from build123d import *

# Parameters (mm, degrees)
SKETCH_1_R      = 12.5
EXTRUDE_1_DEPTH = 4


with BuildPart() as part:
    # 草图1 → 凸台-拉伸1 (new, symmetric)
    with BuildSketch(Plane(origin=(0, 0, 0), x_dir=(1, 0, 0), z_dir=(0, 1, 0))):
        Polygon((-75, 99.709683748), (75, 99.709683748), (119.42074844, 45.609802898), (85, -37.547951261), (-85, -37.547951261), (-119.42074844, 45.609802898), align=None)
        with Locations(Location((-95.730005712, 40.398538957, 0), (0, 0, 270))):
            Circle(SKETCH_1_R, mode=Mode.SUBTRACT)
        with Locations(Location((-39, 80.971951072, 0), (0, 0, 270))):
            Circle(SKETCH_1_R, mode=Mode.SUBTRACT)
        with Locations(Location((-39, -20.275462647, 0), (0, 0, 270))):
            Circle(SKETCH_1_R, mode=Mode.SUBTRACT)
        with Locations(Location((39, -20.275462647, 0), (0, 0, 90))):
            Circle(SKETCH_1_R, mode=Mode.SUBTRACT)
        with Locations(Location((39, 80.971951072, 0), (0, 0, 90))):
            Circle(SKETCH_1_R, mode=Mode.SUBTRACT)
        with Locations(Location((95.730005712, 40.398538957, 0), (0, 0, 90))):
            Circle(SKETCH_1_R, mode=Mode.SUBTRACT)
    extrude(amount=EXTRUDE_1_DEPTH, both=True)


solid = part.part
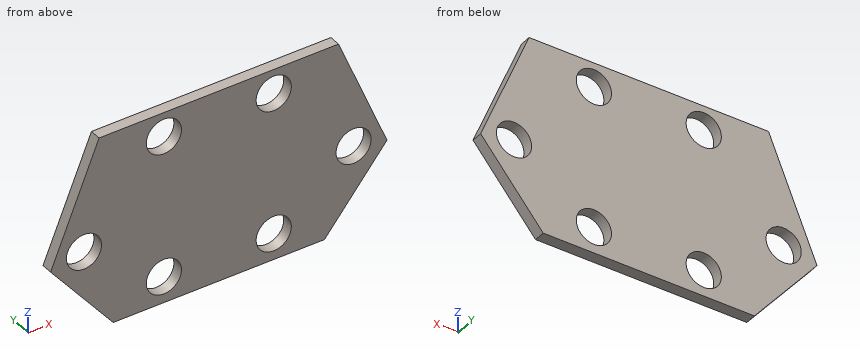
The model under review builds one solid part; all positions refer to its coordinate system, in mm. Give positions to 0.01 mm unless a question says otherwise; leave off trailing zeros. Write each loop counter-clockwise with the first axis right and the second up, starting at its lowest first coordinate (ties: lowest second). Pieces come first, ordered by that corner, then holes.
1. Add section A-A, the plane y = -2. Write out the cut boundary in (x, z).
2. Add section D-D, the plane z = -21. Write out the cut boundary in (x, y), plus the area to 3 significant figures.
3. For P1, Ø4, axis at y = 1.5, z = -33.5, coming from the +X side; P2, Ø3, axis at y = 1, z = -8.5, coming from the +X side, all flat-tipped, find the tip position at first contact; note any pin that passes through.
4. Add section B-B, the plane x = 39. Write out the cut boundary in (y, z).
5. Add section C-C, the plane x = 88.5. Write out the cut boundary in (y, z), plus the area to 3 significant figures.
6. Wall thickness on L1, parallel to Z at x = 39, y = -1.75; L2, parallel to Z at x = 27.5, y = -2.5; L3, parallel to X at y = 0.5, z = -74: over which ranges is each line inside the solid? List them lowest first.
Worked answers:
1. outline: (-119.42, -45.61) - (-75, -99.71) - (75, -99.71) - (119.42, -45.61) - (85, 37.55) - (-85, 37.55) - close; hole circle Ø25 at (-95.73, -40.4); hole circle Ø25 at (-39, -80.97); hole circle Ø25 at (-39, 20.28); hole circle Ø25 at (39, -80.97); hole circle Ø25 at (39, 20.28); hole circle Ø25 at (95.73, -40.4)
2. outline: (-109.23, -4) - (109.23, -4) - (109.23, 4) - (-109.23, 4) - close
2. area: 1,750 mm2
3. P1: stops at x = 115.24
3. P2: stops at x = 104.68
4. outline: (-4, -99.71) - (4, -99.71) - (4, -93.47) - (-4, -93.47) - close; (-4, -68.47) - (4, -68.47) - (4, 7.78) - (-4, 7.78) - close; (-4, 32.78) - (4, 32.78) - (4, 37.55) - (-4, 37.55) - close
5. outline: (-4, -83.27) - (4, -83.27) - (4, -50.6) - (-4, -50.6) - close; (-4, -30.2) - (4, -30.2) - (4, 29.09) - (-4, 29.09) - close
5. area: 736 mm2
6. L1: z = -99.71 to -93.47, -68.47 to 7.78, 32.78 to 37.55
6. L2: z = -99.71 to -85.87, -76.07 to 15.38, 25.17 to 37.55
6. L3: x = -96.11 to -49.38, -28.62 to 28.62, 49.38 to 96.11
